Here's the drawing with two shaded views (mm, measured from the low corner). I have some questions. A direction names the side the tool comes from. Coordinates: 2 decimals unless noted, no trailing zeros. Loops run counter-clockwise (first coordinate to the right, second up) from the corner with the lowest first, then second, coordinate; pieces in that order, holes last.
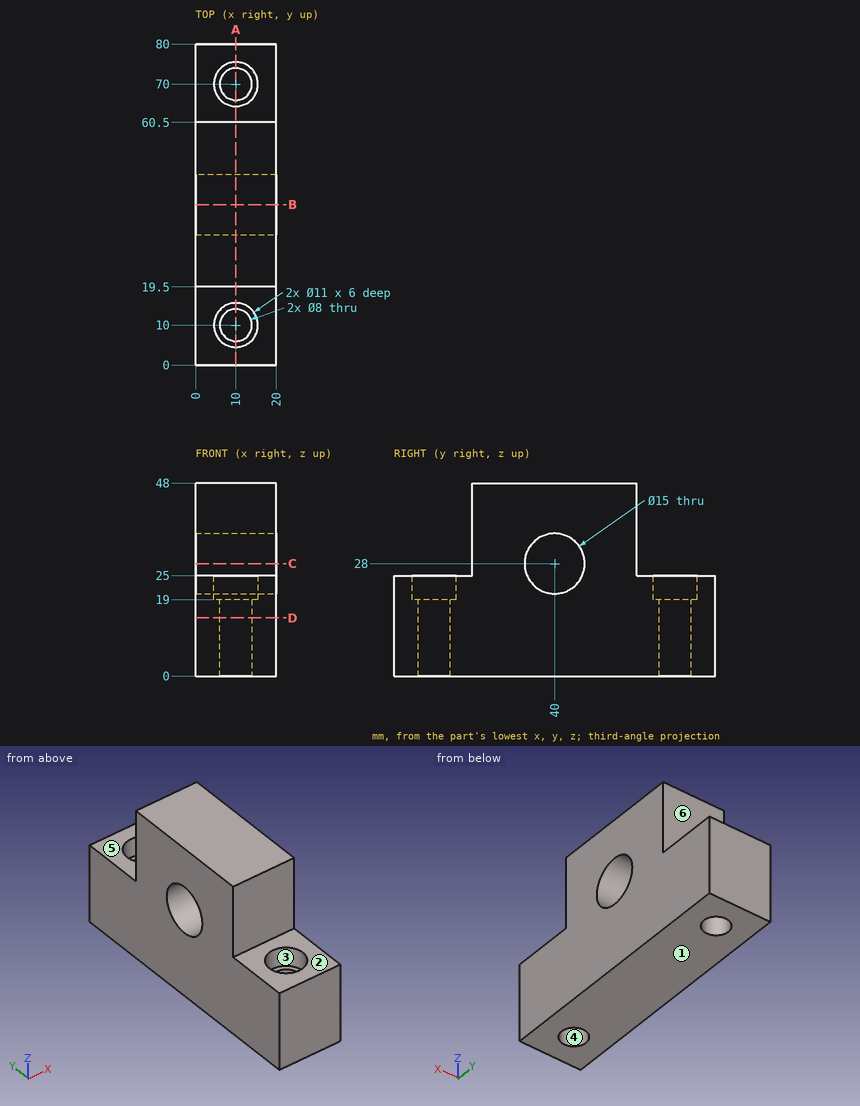
(1) I want a section at B-B on y = 40. Write out the boundary of the cut face in (x, z), then the cut area to 3 significant figures.
Check values:
outline: (0, 0) - (20, 0) - (20, 20.5) - (0, 20.5) - close; (0, 35.5) - (20, 35.5) - (20, 48) - (0, 48) - close
area: 660 mm2
(2) If I drill on probe 1 along Y at (x, z) = (10, 9.5); probe 2 along Y at (x, z) = (10, 22.65); probe 3 along Z at (x, y) = (4.25, 17.5), over which ranges is the centre line in solid material (lowest first)?
Check values:
probe 1: y = 0 to 6, 14 to 66, 74 to 80
probe 2: y = 0 to 4.5, 15.5 to 34.74, 45.26 to 64.5, 75.5 to 80
probe 3: z = 0 to 25
(3) I want a section at C-C on z = 28. Write out the boundary of the cut face in (x, y).
Check values:
outline: (0, 19.5) - (20, 19.5) - (20, 32.5) - (0, 32.5) - close; (0, 47.5) - (20, 47.5) - (20, 60.5) - (0, 60.5) - close
(4) I want a section at D-D on z = 14.5. Write out the boundary of the cut face in (x, y).
Check values:
outline: (0, 0) - (20, 0) - (20, 80) - (0, 80) - close; hole circle Ø8 at (10, 10); hole circle Ø8 at (10, 70)
(5) Which directions (+Z, -Z, +X, -X, +Y, -Y) give clear straight access to the entire face, cutting with the end or side of a thin tool? Please do the marked faces 1, 2 and 3.
Check values:
face 1: -Z, +X, -X, +Y, -Y
face 2: +Z, +X, -X, -Y
face 3: +Z
(6) I'm going to push flat-ended pins straight in: pin 1 (5 mm diameter, centred on x = 10, y = 10, fed in from -Z); pin 2 (6 mm diameter, centred on x = 11, z = 42, fed in from -Y); pin 3 (1 mm diameter, centred on x = 17, y = 30.5, fed in from -Z); pin 4 (5 mm diameter, centred on x = 2.5, z = 33.5, fed in from +Y). Where does each tip first touch, or does it pass through?
Check values:
pin 1: passes through
pin 2: stops at y = 19.5
pin 3: stops at z = 0
pin 4: stops at y = 60.5
(7) I want a section at A-A on x = 10. Write out the boundary of the cut face in (y, z), then the cut area to 3 significant figures.
Check values:
outline: (0, 0) - (6, 0) - (6, 19) - (4.5, 19) - (4.5, 25) - (0, 25) - close; (14, 0) - (66, 0) - (66, 19) - (64.5, 19) - (64.5, 25) - (60.5, 25) - (60.5, 48) - (19.5, 48) - (19.5, 25) - (15.5, 25) - (15.5, 19) - (14, 19) - close; (74, 0) - (80, 0) - (80, 25) - (75.5, 25) - (75.5, 19) - (74, 19) - close; hole circle Ø15 at (40, 28)
area: 2,330 mm2
(8) If we mould it in two halves opening along Y, with no side actions, what happens to the marked faces 4, 5 and 6? For each: released by +Y, released by -Y, zero draft, split by the parting line, or undercut.
Check values:
face 4: undercut
face 5: zero draft
face 6: released by +Y
